Build history of the part. All positions in model axes, mm. Round coordinates to 2 decimals unless told otherwise and drop trailing zeros. Order: outer loops, then holes, each group sorted by start corner. A loop starts at its lowest first (then second) coordinate and runs counter-clockwise, first axis right, second up. Notation, with made-up numbers: (-34.5, -32.75) -> (-3.5, -32.75) arc R8 ccw to (-3.5, -22.75) -> close; hole circle Ø9 at (-36, 44.25). An arc over 180 degrees is marked (long way). Use a Markdown table: item, result. Add a question column.
Item 1: Probe L1, parallel to Y at x = -63, z = -2.9; L2, parallel to Y at x = -61.5, z = -2.5; L3, parallel to X at y = -33, z = -1.25. List the from-to ranges inside material, lowest first.
Item 2: Pin check, flat tips, straight feed: pin 1 (5 mm diameter, centred on x = 0, y = 71.5, fed in from -Z); pin 2 (1.5 mm diameter, centred on y = 72.5, z = -2, fed in from +X); pin 3 (1.5 mm diameter, centred on x = 108.5, z = -1.5, fed in from +Y); pin 4 (1.5 mm diameter, centred on x = -80.5, z = -1, fed in from -Y). Stop position of each tip, or through.
Item 3: Slice it at C-C, the plane z = -0.5. State how many separate pieces and enclosed holes the cut face has, plus the area to 3 significant figures.
Item 4: Slice it at B-B, the plane y = -59.75. Give the cut face in (x, z), plus the area to 3 significant figures.
Item 5: Slice it at A-A, the plane x = -107.5. Give the cut face in (y, z), plus the area to 3 significant figures.
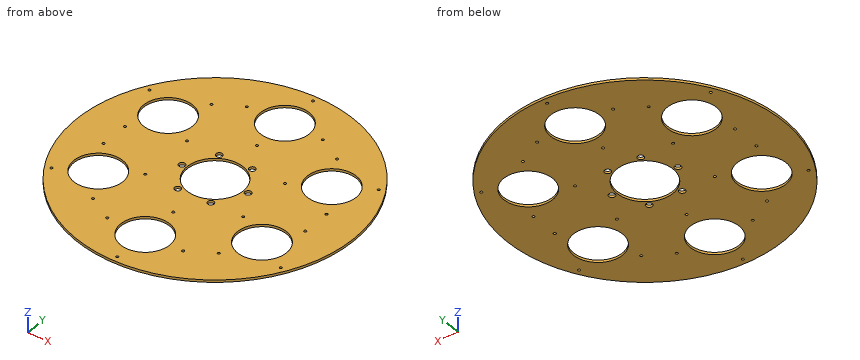
from build123d import *

# Parameters (mm, degrees)
SKETCH1_R           = 175
SKETCH1_R_2         = 35.5
SKETCH1_R_3         = 31
BOSS_EXTRUDE1_DEPTH = 3
SKETCH2_R           = 1.6
CUT_EXTRUDE1_DEPTH  = 3
SKETCH3_R           = 4
CUT_EXTRUDE2_DEPTH  = 3


with BuildPart() as part:
    # Sketch1 → Boss-Extrude1 (new body)
    with BuildSketch(Plane.XY):
        Circle(SKETCH1_R)
        Circle(SKETCH1_R_2, mode=Mode.SUBTRACT)
        with Locations((0, 119.5)):
            Circle(SKETCH1_R_3, mode=Mode.SUBTRACT)
        with Locations((103.490035752, 59.75)):
            Circle(SKETCH1_R_3, mode=Mode.SUBTRACT)
        with Locations((103.490035752, -59.75)):
            Circle(SKETCH1_R_3, mode=Mode.SUBTRACT)
        with Locations((0, -119.5)):
            Circle(SKETCH1_R_3, mode=Mode.SUBTRACT)
        with Locations((-103.490035752, -59.75)):
            Circle(SKETCH1_R_3, mode=Mode.SUBTRACT)
        with Locations((-103.490035752, 59.75)):
            Circle(SKETCH1_R_3, mode=Mode.SUBTRACT)
    extrude(amount=-BOSS_EXTRUDE1_DEPTH)

    # Sketch2 → Cut-Extrude1 (cut)
    with BuildSketch(Plane.XY):
        with Locations((0, 71.5)):
            Circle(SKETCH2_R)
        with Locations((-48, 119.5)):
            Circle(SKETCH2_R)
        with Locations((0, 167.5)):
            Circle(SKETCH2_R)
        with Locations((48, 119.5)):
            Circle(SKETCH2_R)
        with Locations((61.920816371, 35.75)):
            Circle(SKETCH2_R)
        with Locations((79.490035752, 101.319219382)):
            Circle(SKETCH2_R)
        with Locations((145.059255134, 83.75)):
            Circle(SKETCH2_R)
        with Locations((127.490035752, 18.180780618)):
            Circle(SKETCH2_R)
        with Locations((61.920816371, -35.75)):
            Circle(SKETCH2_R)
        with Locations((127.490035752, -18.180780618)):
            Circle(SKETCH2_R)
        with Locations((145.059255134, -83.75)):
            Circle(SKETCH2_R)
        with Locations((79.490035752, -101.319219382)):
            Circle(SKETCH2_R)
        with Locations((0, -71.5)):
            Circle(SKETCH2_R)
        with Locations((48, -119.5)):
            Circle(SKETCH2_R)
        with Locations((0, -167.5)):
            Circle(SKETCH2_R)
        with Locations((-48, -119.5)):
            Circle(SKETCH2_R)
        with Locations((-61.920816371, -35.75)):
            Circle(SKETCH2_R)
        with Locations((-79.490035752, -101.319219382)):
            Circle(SKETCH2_R)
        with Locations((-145.059255134, -83.75)):
            Circle(SKETCH2_R)
        with Locations((-127.490035752, -18.180780618)):
            Circle(SKETCH2_R)
        with Locations((-61.920816371, 35.75)):
            Circle(SKETCH2_R)
        with Locations((-127.490035752, 18.180780618)):
            Circle(SKETCH2_R)
        with Locations((-145.059255134, 83.75)):
            Circle(SKETCH2_R)
        with Locations((-79.490035752, 101.319219382)):
            Circle(SKETCH2_R)
    extrude(amount=-CUT_EXTRUDE1_DEPTH, mode=Mode.SUBTRACT)

    # Sketch3 → Cut-Extrude2 (cut)
    with BuildSketch(Plane.XY):
        with Locations((-21.081787365, 35.74644376)):
            Circle(SKETCH3_R)
        with Locations((20.416434709, 36.130585295)):
            Circle(SKETCH3_R)
        with Locations((41.498222074, 0.384141535)):
            Circle(SKETCH3_R)
        with Locations((-41.498222074, -0.384141535)):
            Circle(SKETCH3_R)
        with Locations((-20.416434709, -36.130585295)):
            Circle(SKETCH3_R)
        with Locations((21.081787365, -35.74644376)):
            Circle(SKETCH3_R)
    extrude(amount=-CUT_EXTRUDE2_DEPTH, mode=Mode.SUBTRACT)


solid = part.part
Check sheet entries:
| question | item | result |
|---|---|---|
| 1 | L1 | -163.27 to -36.93, -34.57 to 34.57, 36.93 to 163.27 |
| 1 | L2 | -163.84 to -37.29, -34.21 to 34.21, 37.29 to 163.84 |
| 1 | L3 | -171.86 to -119.16, -87.82 to -22.91, -17.93 to -13.09, 13.09 to 18.17, 23.99 to 87.82, 119.16 to 171.86 |
| 2 | pin 1 | z = -3 |
| 2 | pin 2 | x = 159.61 |
| 2 | pin 3 | y = 137.89 |
| 2 | pin 4 | y = -155.77 |
| 3 | separate pieces | 1 |
| 3 | enclosed holes | 37 |
| 3 | area | 73,600 mm2 |
| 4 | outline | (-164.48, -3) -> (-134.49, -3) -> (-134.49, 0) -> (-164.48, 0) -> close; (-72.49, -3) -> (72.49, -3) -> (72.49, 0) -> (-72.49, 0) -> close; (134.49, -3) -> (164.48, -3) -> (164.48, 0) -> (134.49, 0) -> close |
| 4 | area | 615 mm2 |
| 5 | outline | (-138.09, -3) -> (-90.49, -3) -> (-90.49, 0) -> (-138.09, 0) -> close; (-29.01, -3) -> (29.01, -3) -> (29.01, 0) -> (-29.01, 0) -> close; (90.49, -3) -> (138.09, -3) -> (138.09, 0) -> (90.49, 0) -> close |
| 5 | area | 460 mm2 |
